from build123d import *

# Parameters (mm, degrees)
SKETCH_4_R          = 1.85
CUT_EXTRUDE_1_DEPTH = 20
SKETCH_5_R          = 1.85
CUT_EXTRUDE_2_DEPTH = 84.417206125


with BuildPart() as part:
    # Эскиз1 → По сечениям1 section 0
    with BuildSketch(Plane(origin=(0, 0, 0), x_dir=(1, 0, 0), z_dir=(0, 1, 0))):
        with BuildLine():
            Line((-75.529594285, -33.966316269), (75.529594285, -33.966316269))
            Line((75.529594285, -33.966316269), (75.529594285, 33.966316269))
            Line((75.529594285, 33.966316269), (-75.529594285, 33.966316269))
            Line((-75.529594285, 33.966316269), (-75.529594285, -33.966316269))
        make_face()
    # Эскиз2 → По сечениям1 section 1
    with BuildSketch(Plane(origin=(0, 10, 0), x_dir=(1, 0, 0), z_dir=(0, 1, 0))):
        with BuildLine():
            Line((65.529594285, -23.966316269), (65.529594285, 23.966316269))
            Line((65.529594285, 23.966316269), (-65.529594285, 23.966316269))
            Line((-65.529594285, 23.966316269), (-65.529594285, -23.966316269))
            Line((-65.529594285, -23.966316269), (65.529594285, -23.966316269))
        make_face()
    loft()

    # Эскиз4 → Вырез-Вытянуть1 (cut)
    with BuildSketch(Plane.XY.offset(33.966316269)):
        with Locations((-60.529594285, 5)):
            Circle(SKETCH_4_R)
        with Locations(Location((60.529594285, 5, 0), (0, 0, 270))):
            Circle(SKETCH_4_R)
    cut_extrude_1 = extrude(amount=-CUT_EXTRUDE_1_DEPTH, mode=Mode.SUBTRACT)

    # Зеркальное отражение1: Вырез-Вытянуть1 across plane
    add(cut_extrude_1.mirror(Plane.XY), mode=Mode.SUBTRACT)

    # Эскиз5 → Вырез-Вытянуть2 (cut, through all)
    with BuildSketch(Plane.XZ):
        with Locations(Location((-70.529594285, 8.966316269, 0), (0, 0, 270))):
            Circle(SKETCH_5_R)
        with Locations(Location((-70.529594285, -8.966316269, 0), (0, 0, 180))):
            Circle(SKETCH_5_R)
        with Locations(Location((70.529594285, -8.966316269, 0), (0, 0, 270))):
            Circle(SKETCH_5_R)
        with Locations((70.529594285, 8.966316269)):
            Circle(SKETCH_5_R)
    extrude(amount=-CUT_EXTRUDE_2_DEPTH, mode=Mode.SUBTRACT)


solid = part.part
Part model, mm, in its own coordinate system. A direction names the side the tool comes from. Give positions to 0.01 mm unless a question says otherwise; leave off trailing zeros. One line per question, with ' | ' between items.
1. Band-saw the part on A-A on y = 1.5. Give the number of separate pieces and of enclosed holes in the cut face, then the cut area to 3 significant figures.
Filled in:
separate pieces: 1 | enclosed holes: 4 | area: 9,570 mm²
2. Drop flat-ended pins along their axis: P1, Ø1.5, axis at y = 7.5, z = 4, coming from the -X side; P2, Ø1, axis at y = 8.5, z = 13.5, coming from the -X side; P3, Ø5, axis at x = -70.53, z = -8.97, coming from the -Y side; P4, Ø4, axis at x = 60, y = 4.5, coming from the +Z side. Give the stop position or say it passes through.
Filled in:
P1: x = -68.78 | P2: x = -67.53 | P3: y = 0 | P4: z = 31.47
3. Drill centre lines: probe 1 along X at (y, z) = (0.5, 8); probe 2 along X at (y, z) = (5, -18.5); probe 3 along X at (y, z) = (3, -28). Where is each one in solid material? Low to high.
Filled in:
probe 1: -75.03 to -72.11, -68.95 to 68.95, 72.11 to 75.03 | probe 2: -70.53 to -62.38, -58.68 to 58.68, 62.38 to 70.53 | probe 3: -72.53 to 72.53
4. Pull direction Z, two halves, no side cores. Call faces 4 (the face through (-60.931, 3.194, 22.509)), 5 (the face through (68.68, 2.62, 9.05)), 6 (the face through (68.724, 2.616, -8.565)), 7 (the face through (-61, 5, -13.966)): +Z half, -Z half, draft (parallel to the pull), parting line (faces both ways), or undercut.
Filled in:
face 4: draft | face 5: undercut | face 6: undercut | face 7: -Z half
5. Which spindle directions (+Z, -Z, +X, -X, +Y, -Y) get a long thin tool onto all of the face, cutting with end or side? Do faces 1 (the face through (59.8, 3.3, -20.6)), 2 (the face through (-1, 0, 1)), 3 (the face through (-61, 5, 13.966)). Say none if no direction does.
Filled in:
face 1: -Z | face 2: +Z, -Z, +X, -X, -Y | face 3: +Z
